CAD build for the part. Positions are in the model's coordinates, mm. A direction names the side the tool comes from. Round coordinates to 2 decimals unless told otherwise and drop trailing zeros. Order: outer loops, then holes, each group sorted by start corner. A loop starts at its lowest first (then second) coordinate and runs counter-clockwise, first axis right, second up. Notation, with made-up numbers: M 12,25.5 L 42,25.5 A18 cw 42,41.5 Z; hole C 7,-24.75 d7. An arc over 180 degrees is marked long. Put each result on its own line as item: value.
```python
from build123d import *

# Parameters (mm, degrees)
F0_W      = 973
F0_H      = 566
F1_DEPTH  = 31
F2_W      = 789
F2_H      = 466
F3_DEPTH  = 41
F4_W      = 36.994547
F4_H      = 11.94332
F5_DEPTH  = 5
F6_W      = 930
F6_H      = 523
F7_DEPTH  = 1
F8_R      = 3
F9_DEPTH  = 43
F11_DEPTH = 881.001


with BuildPart() as f1:
    # F0 (on Front) → F1 (new body)
    with BuildSketch(Plane.XZ):
        Rectangle(F0_W, F0_H)
    extrude(amount=F1_DEPTH)

    # F2 (on face) → F3 (join)
    with BuildSketch(Plane(origin=(0, 0, 0), x_dir=(-1, 0, 0), z_dir=(0, 1, 0))):
        with Locations((0, 32)):
            Rectangle(F2_W, F2_H)
    extrude(amount=F3_DEPTH)

    # F4 (on face) → F5 (cut)
    with BuildSketch(Plane(origin=(0, 0, -201), x_dir=(1, 0, 0), z_dir=(0, 0, -1))):
        with Locations((210.368886, -20.5)):
            Rectangle(F4_W, F4_H)
    extrude(amount=-F5_DEPTH, mode=Mode.SUBTRACT)

    # F6 (on face) → F7 (cut)
    with BuildSketch(Plane.XZ.offset(31)):
        Rectangle(F6_W, F6_H)
    extrude(amount=-F7_DEPTH, mode=Mode.SUBTRACT)

    # F8 (on face) → F9 (join)
    with BuildSketch(Plane(origin=(0, 0, 0), x_dir=(-1, 0, 0), z_dir=(0, 1, 0))):
        with Locations((-150, 150)):
            Circle(F8_R)
        with Locations((150, 150)):
            Circle(F8_R)
        with Locations((-150, -150)):
            Circle(F8_R)
        with Locations((150, -150)):
            Circle(F8_R)
    extrude(amount=F9_DEPTH)

    # F10 (on face) → F11 (cut, through all)
    with BuildSketch(Plane.YZ.offset(394.5)):
        Polygon((41, 265), (0, 265), (31, 248), (41, 203), align=None)
    extrude(amount=-F11_DEPTH, mode=Mode.SUBTRACT)


solid = f1.part
```
Item 1: Probe line 1 along X through (y, z) = (6.5, 99); line 2 along Y through (x, z) = (365.5, -186.5); line 3 along Y through (x, z) = (-404, -58). List the from-to ranges inside material, lowest first. Write a range as [from, to].
Answers below:
line 1: [-394.5, 394.5]
line 2: [-30, 41]
line 3: [-30, 0]
Item 2: Pin check, flat tips, straight feed: P1, Ø1, axis at x = -325.5, z = 153.5, coming from the -Y side; P2, Ø12.5, axis at y = 22, z = 126, coming from the +X side; P3, Ø2.5, axis at y = 22.5, z = -198, coming from the -X side. Stop position of each tip, or through.
Answers below:
P1: y = -30
P2: x = 394.5
P3: x = -394.5
Item 3: Mould opens along X. For faces 1 (the flat face through (-394.5, 20, 29)), 2 (the flat face through (394.5, 20, 29)), 3 (the flat face through (-2, 0, -208)), 4 (the flat face through (-7, -30, 4)) say: pulls with the +X half, pulls with the -X half, needs draft (parallel to the pull), parting line crosses it, or undercut.
Answers below:
face 1: pulls with the -X half
face 2: pulls with the +X half
face 3: needs draft
face 4: undercut
Item 4: Tool access for faces 5 (the flat face through (6, 20, -201)), 6 (the flat face through (-7, -15, 283)): list every direction of +Z, -Z, +X, -X, +Y, -Y with a clear straight run to the whole face (end or side of a thin tool).
Answers below:
face 5: -Z, +X, -X, +Y
face 6: +Z, +X, -X, +Y, -Y
Item 5: Band-saw the part on A-A on x = -299. Give the cut face in (y, z), and give its area (3 significant figures).
Answers below:
outline: M -31,-283 L 0,-283 L 0,-201 L 41,-201 L 41,203 L 31,248 L 0,265 L 0,283 L -31,283 L -31,261.5 L -30,261.5 L -30,-261.5 L -31,-261.5 Z
area: 35,500 mm²
